Geometry check sheet. Reference: the model listing, model coordinates, mm. Coordinates: 2 decimals unless noted, no trailing zeros. Write each loop counter-clockwise with the first axis right and the second up, starting at its lowest first coordinate (ties: lowest second). Pieces come first, ordered by that corner, then holes. Notation, with made-up numbers: (-27, 85) -> (31, 85) arc R29 cw to (31, 124) -> close; hole circle Ø9 at (42.5, -28). An arc over 180 degrees is marked (long way). Answer in a Markdown table with one row per item. Add a question column.
1. Cross-section at B-B on z = 5.5. Give the number of separate pieces and of enclosed holes in the cut face, and give its area (3 significant figures).
2. Scan lines: L1, parallel to X at y = 19, z = 3.75; L2, parallel to Z at x = 151, y = 42.5; L3, parallel to X at y = -1, z = 11. Record each from-to range of solid material in increasing order. Write a range as from..to.
3. Depth check by flat-ended pin: P1, Ø3, axis at x = 72.5, y = 64, coming from the +Z side; P2, Ø10, axis at y = 4, z = 8, coming from the +X side; P3, Ø1, axis at x = 41.5, z = 9, coming from the -Y side. Enter the tip coordinate at first touch or a pass-through.
4. Cross-section at A-A on y = 26. Record the cut outline in (x, z).
```python
from build123d import *

# Parameters (mm, degrees)
MODEL_W              = 228.552502
MODEL_H              = 118.27002
MODEL_W_2            = 80.01
MODEL_H_2            = 36.195
BOSS_EXTRUDE3_DEPTH  = 1.5875
SKETCH4_R            = 6.1976
BOSS_EXTRUDE4_DEPTH  = 8.9916
LPATTERN1_COUNT      = 15
LPATTERN1_PITCH      = 12.7
LPATTERN1_COUNT_DIR2 = 2
LPATTERN1_PITCH_DIR2 = 25.4
SKETCH5_R            = 2.9972
BOSS_EXTRUDE5_DEPTH  = 10.9982
SKETCH8_W            = 2.447124678
SKETCH8_H            = 7.642831421
CUT_EXTRUDE1_DEPTH   = 7.0104
LPATTERN2_COUNT      = 15
LPATTERN2_PITCH      = 12.7
LPATTERN2_COUNT_DIR2 = 2
LPATTERN2_PITCH_DIR2 = 25.4
SKETCH6_W            = 10.0076
SKETCH6_H            = 10.0076
BOSS_EXTRUDE6_DEPTH  = 10.9982
LPATTERN3_COUNT      = 3
LPATTERN3_PITCH      = 19.05
LPATTERN3_COUNT_DIR2 = 2
LPATTERN3_PITCH_DIR2 = 19.05
LPATTERN4_COUNT      = 2
LPATTERN4_PITCH      = 19.05
LPATTERN4_COUNT_DIR2 = 2
LPATTERN4_PITCH_DIR2 = 19.05


with BuildPart() as part:
    # Model → Boss-Extrude3 (new body)
    with BuildSketch(Plane.XY):
        with Locations((114.276251, 46.773846)):
            Rectangle(MODEL_W, MODEL_H)
        with Locations((70.485, 15.875)):
            Rectangle(MODEL_W_2, MODEL_H_2, mode=Mode.SUBTRACT)
    extrude(amount=BOSS_EXTRUDE3_DEPTH)

    # Sketch4 → Boss-Extrude4 (add)
    with BuildSketch(Plane.XY.offset(1.5875)):
        with Locations(Location((25.4, 92.71, 0), (0, 0, 180))):
            Circle(SKETCH4_R)
    boss_extrude4 = extrude(amount=BOSS_EXTRUDE4_DEPTH)

    # LPattern1: Boss-Extrude4 15 × 2, 15 skipped
    with Locations(*[(i * LPATTERN1_PITCH, -j * LPATTERN1_PITCH_DIR2, 0) for i in range(LPATTERN1_COUNT) for j in range(LPATTERN1_COUNT_DIR2) if (i, j) not in ((0, 0), (0, 1), (1, 0), (2, 1), (3, 0), (4, 1), (5, 0), (6, 1), (7, 0), (8, 1), (9, 0), (10, 1), (11, 0), (12, 1), (13, 0), (14, 1))]):
        add(boss_extrude4)

    # Sketch5 → Boss-Extrude5 (add)
    with BuildSketch(Plane.XY.offset(10.5791)):
        with Locations((25.4, 92.71)):
            Circle(SKETCH5_R)
    boss_extrude5 = extrude(amount=BOSS_EXTRUDE5_DEPTH)

    # Sketch8 → Cut-Extrude1 (cut)
    with BuildSketch(Plane.XY.offset(21.5773)):
        with Locations((22.677837661, 92.551291415)):
            Rectangle(SKETCH8_W, SKETCH8_H)
    cut_extrude1 = extrude(amount=-CUT_EXTRUDE1_DEPTH, mode=Mode.SUBTRACT)

    # LPattern2: Boss-Extrude5, Cut-Extrude1 15 × 2, 15 skipped
    with Locations(*[(i * LPATTERN2_PITCH, -j * LPATTERN2_PITCH_DIR2, 0) for i in range(LPATTERN2_COUNT) for j in range(LPATTERN2_COUNT_DIR2) if (i, j) not in ((0, 0), (0, 1), (1, 0), (2, 1), (3, 0), (4, 1), (5, 0), (6, 1), (7, 0), (8, 1), (9, 0), (10, 1), (11, 0), (12, 1), (13, 0), (14, 1))]):
        add(boss_extrude5)
        add(cut_extrude1, mode=Mode.SUBTRACT)

    # Sketch6 → Boss-Extrude6 (add)
    with BuildSketch(Plane.XY.offset(1.5875)):
        with Locations((148.965412, 16.383)):
            Rectangle(SKETCH6_W, SKETCH6_H)
    boss_extrude6 = extrude(amount=BOSS_EXTRUDE6_DEPTH)

    # LPattern3: Boss-Extrude6 3 × 2, 3 skipped
    with Locations(*[(i * LPATTERN3_PITCH, -j * LPATTERN3_PITCH_DIR2, 0) for i in range(LPATTERN3_COUNT) for j in range(LPATTERN3_COUNT_DIR2) if (i, j) not in ((0, 0), (0, 1), (1, 0), (2, 1))]):
        add(boss_extrude6)

    # LPattern4: Boss-Extrude6 2 × 2, 2 skipped
    with Locations(*[(j * LPATTERN4_PITCH_DIR2, i * LPATTERN4_PITCH, 0) for i in range(LPATTERN4_COUNT) for j in range(LPATTERN4_COUNT_DIR2) if (i, j) not in ((0, 0), (0, 1), (1, 0))]):
        add(boss_extrude6)


solid = part.part
```
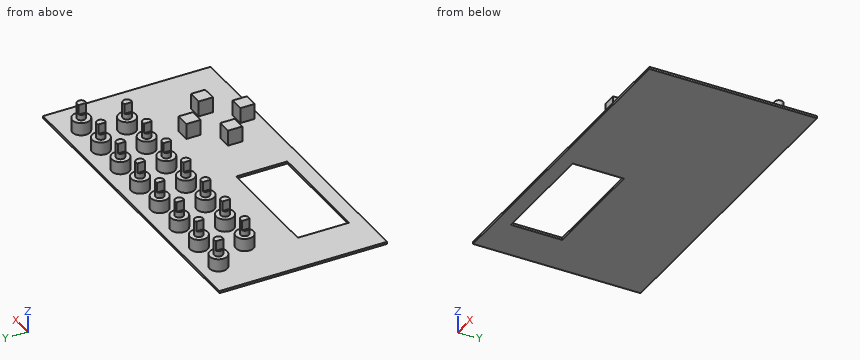
Results found:
| question | item | result |
|---|---|---|
| 1 | separate pieces | 19 |
| 1 | enclosed holes | 0 |
| 1 | area | 2,210 mm^2 |
| 2 | L1 | x = 143.96..153.97, 182.06..192.07 |
| 2 | L2 | z = 0..1.59 |
| 2 | L3 | x = 163.01..173.02 |
| 3 | P1 | stops at z = 1.59 |
| 3 | P2 | stops at x = 173.02 |
| 3 | P3 | stops at y = 61.83 |
| 4 | outline | (0, 0) -> (30.48, 0) -> (30.48, 1.59) -> (0, 1.59) -> close; (110.49, 0) -> (228.55, 0) -> (228.55, 1.59) -> (110.49, 1.59) -> close |
